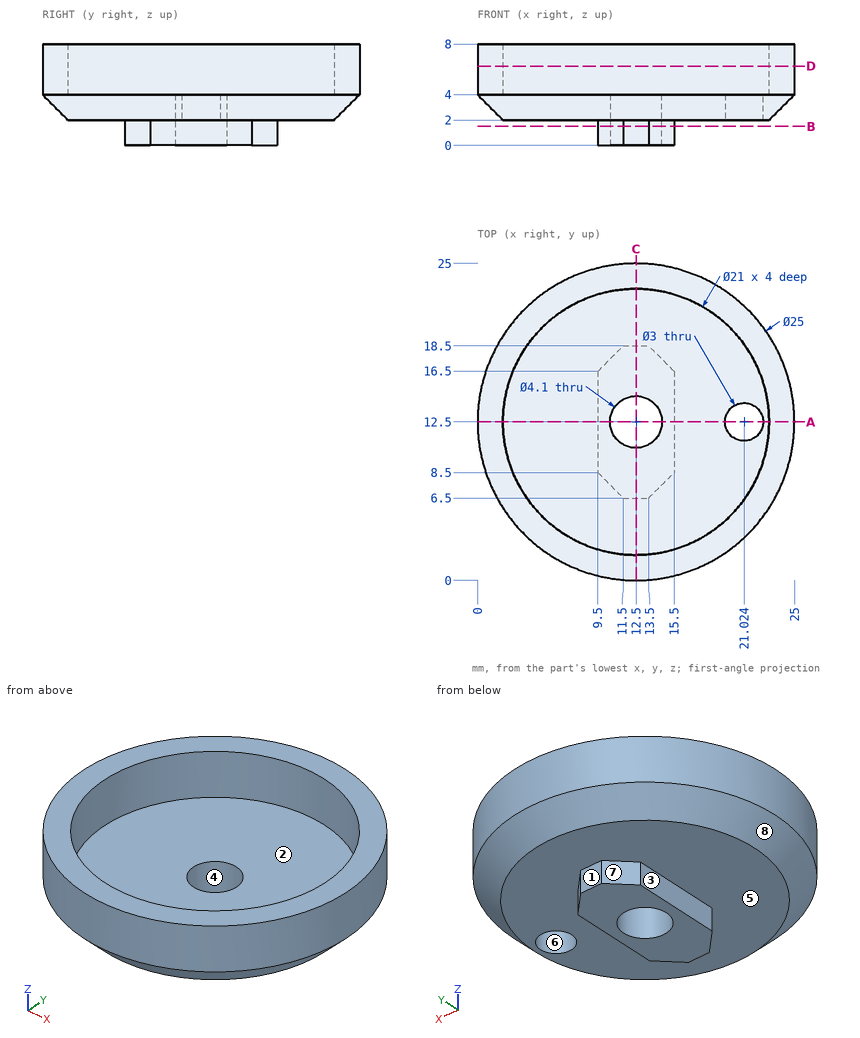
Verification items for this drawing (mm, ordinates from the low corner). A direction names the side the tool comes from. Give positions to 0.01 mm unless a question says otherwise; leave off trailing zeros. Loops run counter-clockwise (first coordinate to the right, second up) from the corner with the lowest first, then second, coordinate; pieces in that order, holes last. Notation, with made-up numbers: M 67,57.5 L 86,57.5 A15 cw 86,81.5 Z; hole C 4,20 d7. An arc over 180 degrees is marked long. Return JSON: item names as keys, results as strings. Group by question number.
1. Thickness scan on L1, parallel to Z at x = 8.5, y = 20.5; L2, parallel to Y at x = 19, z = 6 (1 decimal); L3, parallel to X at y = 10.75, z = 7.75. Record the ranges inside material, lowest first.
2. Go/stop test with flat-tipped pins: pin 1 (5 mm diameter, centred on x = 21.02, y = 12.5, fed in from -Z); pin 2 (0.6 mm diameter, centred on y = 14.5, z = 1, fed in from +X); pin 3 (4 mm diameter, centred on x = 15, z = 3.5, fed in from +Y). Record where each tip stops, or that it passes through.
3. Cross-section at C-C on x = 12.5. Record the boundary of the cut face in (y, z).
4. Tool access check on the marked faces 1, 2, 3, 4 and 5. Record the directions out of +Z, -Z, +X, -X, +Y, -Y that give a thin tool (end or side, any length) a straight path to the whole face; none if there is none.
5. Cross-section at D-D on z = 6.25. Record the boundary of the cut face in (x, y).
6. Cross-section at A-A on y = 12.5. Record the boundary of the cut face in (x, z).
7. Mould release check, pull along X, two halves, no side actions. Record for the marked faces 6, 7 and 8: released by +X, released by -X, zero draft, split by the parting line, or undercut.
8. Cross-section at B-B on z = 1.5. Record the boundary of the cut face in (x, y), plus the area to 3 significant figures.
Return value:
{
 "1": {"L1": "2 to 4", "L2": "1.8 to 4.3, 20.7 to 23.2", "L3": "0.12 to 2.15, 22.85 to 24.88"},
 "2": {"pin 1": "z = 2", "pin 2": "x = 15.5", "pin 3": "y = 24.99"},
 "3": {"outline": "M 0,4 L 2,2 L 6.5,2 L 6.5,0 L 10.45,0 L 10.45,4 L 2,4 L 2,8 L 0,8 Z; M 14.55,0 L 18.5,0 L 18.5,2 L 23,2 L 25,4 L 25,8 L 23,8 L 23,4 L 14.55,4 Z"},
 "4": {"face 1": "-Z, +X, -X, +Y", "face 2": "+Z", "face 3": "-Z, -X, +Y, -Y", "face 4": "+Z, -Z", "face 5": "-Z"},
 "5": {"outline": "C 12.5,12.5 d25; hole C 12.5,12.5 d21"},
 "6": {"outline": "M 0,4 L 2,2 L 9.5,2 L 9.5,0 L 10.45,0 L 10.45,4 L 2,4 L 2,8 L 0,8 Z; M 14.55,0 L 15.5,0 L 15.5,2 L 19.52,2 L 19.52,4 L 14.55,4 Z; M 22.52,2 L 23,2 L 25,4 L 25,8 L 23,8 L 23,4 L 22.52,4 Z"},
 "7": {"face 6": "undercut", "face 7": "released by -X", "face 8": "split by the parting line"},
 "8": {"outline": "M 9.5,8.5 L 11.5,6.5 L 13.5,6.5 L 15.5,8.5 L 15.5,16.5 L 13.5,18.5 L 11.5,18.5 L 9.5,16.5 Z; hole C 12.5,12.5 d4.1", "area": "50.8 mm^2"}
}
